Build history of the part. All positions in model axes, mm. A direction names the side the tool comes from. Round coordinates to 2 decimals unless told otherwise and drop trailing zeros. Write each loop counter-clockwise with the first axis right and the second up, starting at its lowest first coordinate (ties: lowest second). Pieces come first, ordered by that corner, then holes. Notation, with made-up numbers: (-2, -27.75) -> (20, -27.75) arc R26 ccw to (20, -2.75) -> close; hole circle Ø7 at (77.5, -24). An arc over 180 degrees is marked (long way). Return JSON: item names as keys, results as strings.
from build123d import *

# Parameters (mm, degrees)
SKETCH1_R           = 10
BOSS_EXTRUDE1_DEPTH = 10.7
BOSS_EXTRUDE2_DEPTH = 9


with BuildPart() as part:
    # Sketch1 → Boss-Extrude1 (new body)
    with BuildSketch(Plane(origin=(0, 0, 0), x_dir=(1, 0, 0), z_dir=(0, 1, 0))):
        with Locations(Location((0, 0, 0), (0, 0, 270))):
            Circle(SKETCH1_R)
    extrude(amount=BOSS_EXTRUDE1_DEPTH)

    # Sketch2 → Boss-Extrude2 (add)
    with BuildSketch(Plane(origin=(0, 10.7, 0), x_dir=(1, 0, 0), z_dir=(0, 1, 0))):
        with BuildLine():
            ThreePointArc((-3.377869151, 7.8), (-8.5, 0), (-3.377869151, -7.8))
            Line((-3.377869151, -7.8), (3.377869151, -7.8))
            ThreePointArc((3.377869151, -7.8), (8.5, 0), (3.377869151, 7.8))
            Line((3.377869151, 7.8), (-3.377869151, 7.8))
        make_face()
    extrude(amount=BOSS_EXTRUDE2_DEPTH)


solid = part.part
Q1. Saw through at C-C on y = 16. List the corners of the cut face in (x, z), then the cut area to 3 significant figures.
Verdict:
{"outline": "(-3.38, -7.8) -> (3.38, -7.8) arc R8.5 ccw to (3.38, 7.8) -> (-3.38, 7.8) arc R8.5 ccw to start", "area": "221 mm²"}
Q2. Saw through at D-D on y = 8. List the corners of the cut face in (x, z).
Verdict:
{"outline": "circle Ø20 at (0, 0)"}
Q3. Saw through at A-A on z = 0. List the corners of the cut face in (x, y), then the cut area to 3 significant figures.
Verdict:
{"outline": "(-10, 0) -> (10, 0) -> (10, 10.7) -> (8.5, 10.7) -> (8.5, 19.7) -> (-8.5, 19.7) -> (-8.5, 10.7) -> (-10, 10.7) -> close", "area": "367 mm²"}
Q4. Wall check: L1, parallel to X at y = 8.75, z = -0.25; L2, parallel to Z at x = 1.5, y = 11; L3, parallel to Y at x = 2.5, z = -8. Give the ranges that are in metal, low to high.
Verdict:
{"L1": "x = -10 to 10", "L2": "z = -7.8 to 7.8", "L3": "y = 0 to 10.7"}
Q5. Pin check, flat tips, straight feed: pin 1 Ø6 at (x, y) = (7, 10) entering from +Z; pin 2 Ø8 at (x, y) = (3, 14) entering from +Z; pin 3 Ø1 at (x, y) = (2, 10.5) entering from +Z. Stop position of each tip, or through.
Verdict:
{"pin 1": "stops at z = 9.17", "pin 2": "stops at z = 9.97", "pin 3": "stops at z = 9.89"}
Q6. 3-axis set-ups, long thin cutter, end or side, ignore diameter. For faces 1 (the cylindrical face through (-8.5, 15.1, -0.1)), 2 (the flat face through (0, 10.7, 8)), 3 (the flat face through (0, 15, -7.8)): which of +Z, -Z, +X, -X, +Y, -Y reach the whole face in a straight line?
Verdict:
{"face 1": "-X, +Y", "face 2": "+Y", "face 3": "-Z, +X, -X, +Y"}
Q7. Two-plate mould, pull along Z, no slides. Class faces 4 (the cylindrical face through (8.5, 15.1, 0.1)), 5 (the flat face through (0, 15, 7.8)), 6 (the flat face through (0, 19.7, 0)): +Z half, -Z half, draft (parallel to the pull), parting line (faces both ways), or undercut.
Verdict:
{"face 4": "parting line", "face 5": "+Z half", "face 6": "draft"}
Q8. Saw through at B-B on x = 0. List the corners of the cut face in (y, z).
Verdict:
{"outline": "(0, -10) -> (10.7, -10) -> (10.7, -7.8) -> (19.7, -7.8) -> (19.7, 7.8) -> (10.7, 7.8) -> (10.7, 10) -> (0, 10) -> close"}
